CAD build for the part. Positions are in the model's coordinates, mm. A direction names the side the tool comes from. Coordinates: 2 decimals unless noted, no trailing zeros. Loops run counter-clockwise (first coordinate to the right, second up) from the corner with the lowest first, then second, coordinate; pieces in that order, holes last. Notation, with made-up numbers: (15, 18) -> (50, 18) arc R16 ccw to (50, 38) -> close; hole circle Ø11 at (78.25, 11.25). An arc over 180 degrees is marked (long way). Return JSON: item names as keys, results as strings. Group by question number.
(1) Probe L1, parallel to Y at x = 0.95, z = 0 (3 decimals); L2, parallel to Y at x = 1.45, z = 2; L3, parallel to Z at x = 0.65, y = -5 (3 decimals). List the from-to ranges inside material, lowest first.
(2) Mould opens along Z. For faces 4 (the face through (1, -12.7, 9)), 5 (the face through (0.783, 9.524, 0.138)), 6 (the face through (0.783, -27.873, -10.773)) say: pulls with the +Z half, pulls with the -Z half, needs draft (parallel to the pull), parting line crosses it, or undercut.
(3) Saw through at C-C on y = -49. Write the cut outline in (x, z) (1 decimal).
(4) Flat gauge pin, fed straight in: pin 1 Ø0.5 at (x, z) = (0.5, 8.5) entering from +Y. Where does the tip first touch, or does it go through?
(5) Saw through at D-D on y = -58.5. Write the cut outline in (x, z) (1 decimal).
(6) Saw through at A-A on z = 0. Write the cut outline in (x, y) (1 decimal), then the cut area to 3 significant figures.
(7) Tool access for faces 1 (the face through (0.783, 1.262, 4.006)), 2 (the face through (1, -21, 7.938)), 3 (the face through (0.78, -12.04, -9.61)): list every direction of +Z, -Z, +X, -X, +Y, -Y with a clear straight run to the whole face (end or side of a thin tool).
```python
from build123d import *

# Parameters (mm, degrees)
BOSS_EXTRUDE1_DEPTH  = 1.5875
M8_CLEARANCE_HOLE1_D = 8.4


with BuildPart() as part:
    # Sketch1 → Boss-Extrude1 (new body)
    with BuildSketch(Plane(origin=(0, 0, 0), x_dir=(0, 0, -1), z_dir=(1, 0, 0))):
        with BuildLine():
            Line((-9.525, -65.774638339), (0, -65.774638339))
            Line((0, -65.774638339), (14.2875, -65.774638339))
            Line((14.2875, -65.774638339), (11.553356238, -27.816833207))
            Line((11.553356238, -27.816833207), (9.96995864, -27.930887132))
            Line((9.96995864, -27.930887132), (8.829419389, -12.096911155))
            Line((8.829419389, -12.096911155), (10.412816987, -11.98285723))
            Line((10.412816987, -11.98285723), (9.500385586, 0.684323551))
            ThreePointArc((9.500385586, 0.684323551), (-0.342383043, 9.518844407), (-9.525, 0))
            Line((-9.525, 0), (-9.525, -12.7))
            Line((-9.525, -12.7), (-7.9375, -12.7))
            Line((-7.9375, -12.7), (-7.9375, -28.575))
            Line((-7.9375, -28.575), (-9.525, -28.575))
            Line((-9.525, -28.575), (-9.525, -65.774638339))
        make_face()
    extrude(amount=BOSS_EXTRUDE1_DEPTH)

    # M8 Clearance Hole1 (through all)
    with Locations(Plane(origin=(1.5875, 0, 0), x_dir=(0, 0, -1), z_dir=(1, 0, 0))):
        with Locations((0, 0)):
            Hole(M8_CLEARANCE_HOLE1_D / 2)


solid = part.part
```
Geometry results:
{
 "1": {"L1": "-65.775 to -4.2, 4.2 to 9.525", "L2": "-65.77 to -3.69, 3.69 to 9.31", "L3": "-9.91 to 9.525"},
 "2": {"face 4": "needs draft", "face 5": "parting line crosses it", "face 6": "undercut"},
 "3": {"outline": "(0, -13.1) -> (1.6, -13.1) -> (1.6, 9.5) -> (0, 9.5) -> close"},
 "4": {"pin 1": "y = 4.76"},
 "5": {"outline": "(0, -13.8) -> (1.6, -13.8) -> (1.6, 9.5) -> (0, 9.5) -> close"},
 "6": {"outline": "(0, -65.8) -> (1.6, -65.8) -> (1.6, -4.2) -> (0, -4.2) -> close; (0, 4.2) -> (1.6, 4.2) -> (1.6, 9.5) -> (0, 9.5) -> close", "area": "106 mm²"},
 "7": {"face 1": "+X, -X", "face 2": "+Z, +X, -X", "face 3": "-Z, +X, -X"}
}
